Job drawing, mm, ordinate dimensions from the low corner. One solid piece. A direction names the side the tool comes from. Give positions to 0.01 mm unless a question says otherwise; leave off trailing zeros. Write each loop counter-clockwise with the first axis right and the second up, starting at its lowest first coordinate (ties: lowest second). Pieces come first, ordered by that corner, then holes. Notation, with made-up numbers: M 24.25,71 L 35.25,71 A17 cw 35.25,78 Z; hole C 88.25,81 d5. An arc over 180 degrees is marked long. Use a Markdown table: item, result.
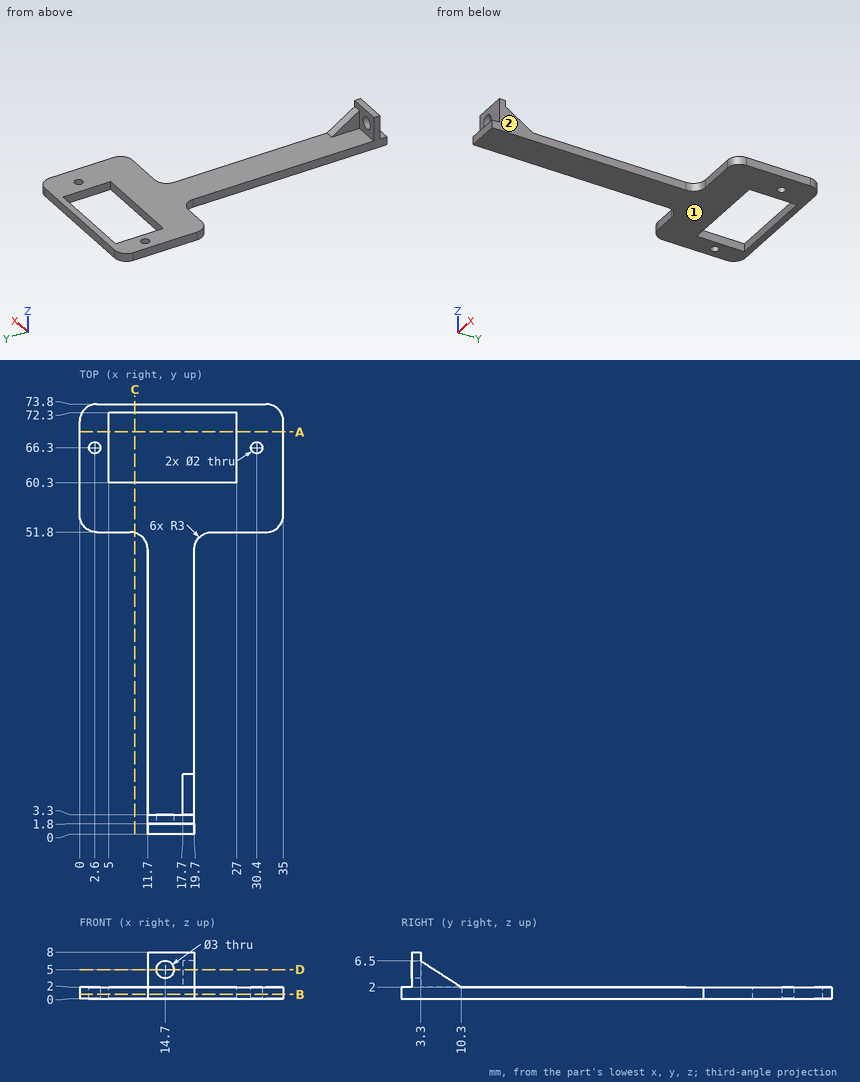
1. Drill centre lines: L1, parallel to X at y = 70.5, z = 1.75; L2, parallel to X at y = 66.3, z = 1.2; L3, parallel to X at y = 2.1, z = 5. Where is each one in solid material? Low to high.
Findings below:
| item | result |
|---|---|
| L1 | 0 to 5, 27 to 35 |
| L2 | 0 to 1.6, 3.6 to 5, 27 to 29.4, 31.4 to 35 |
| L3 | 11.7 to 13.2, 16.2 to 19.7 |
2. Cut at A-A, the plane y = 69. Give the cut face in (x, z), then the cut area to 3 significant figures.
Findings below:
| item | result |
|---|---|
| outline | M 0,0 L 5,0 L 5,2 L 0,2 Z; M 27,0 L 35,0 L 35,2 L 27,2 Z |
| area | 26.0 mm2 |
3. Cut at C-C, the plane x = 9.5. Give the cut face in (y, z), then the cut area to 3 significant figures.
Findings below:
| item | result |
|---|---|
| outline | M 51.69,0 L 60.3,0 L 60.3,2 L 51.69,2 Z; M 72.3,0 L 73.8,0 L 73.8,2 L 72.3,2 Z |
| area | 20.2 mm2 |
4. Cut at D-D, the plane z = 5. Give the cut face in (x, y), then the cut area to 3 significant figures.
Findings below:
| item | result |
|---|---|
| outline | M 11.7,1.8 L 13.2,1.8 L 13.2,3.3 L 11.7,3.3 Z; M 16.2,1.8 L 19.7,1.8 L 19.7,5.63 L 17.7,5.63 L 17.7,3.3 L 16.2,3.3 Z |
| area | 12.2 mm2 |
5. Cut at B-B, the plane z = 0.75. Give the cut face in (x, y).
Findings below:
| item | result |
|---|---|
| outline | M 0,54.8 A3 ccw 3,51.8 L 8.7,51.8 A3 cw 11.7,48.8 L 11.7,0 L 19.7,0 L 19.7,48.8 A3 cw 22.7,51.8 L 32,51.8 A3 ccw 35,54.8 L 35,70.8 A3 ccw 32,73.8 L 3,73.8 A3 ccw 0,70.8 Z; hole C 2.6,66.3 d2; hole M 5,60.3 L 27,60.3 L 27,72.3 L 5,72.3 Z; hole C 30.4,66.3 d2 |
6. Drop flat-ended pins along their axis: P1, Ø10.5, axis at x = 14.5, y = 42, coming from the +Z side; P2, Ø1, axis at x = 26.5, z = 0.5, coming from the -Y side; P3, Ø1.5, axis at x = 11.5, z = 3, coming from the +Y side. Give the stop position or say it passes through.
Findings below:
| item | result |
|---|---|
| P1 | z = 2 |
| P2 | y = 51.8 |
| P3 | y = 3.3 |
7. Tool access for the marked faces 1 and 2: list every direction of +Z, -Z, +X, -X, +Y, -Y with a clear straight run to the whole face (end or side of a thin tool).
Findings below:
| item | result |
|---|---|
| face 1 | -Z, +X, -X, +Y, -Y |
| face 2 | +Z, -Z, +X, -Y |
